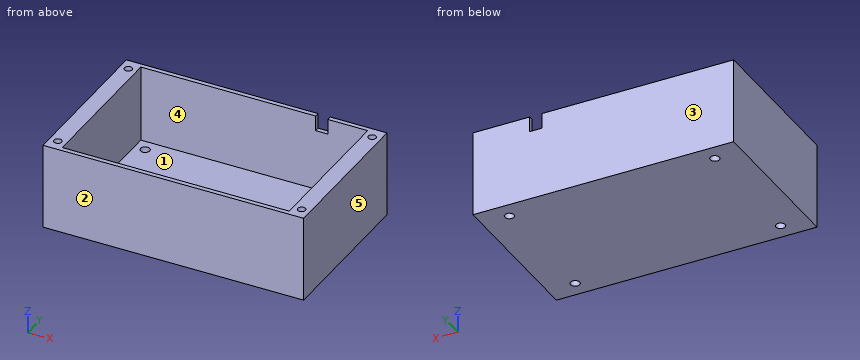
from build123d import *

# Parameters (mm, degrees)
F0_W     = 85
F0_H     = 52
F0_R     = 1.5
F1_DEPTH = 3
F2_W     = 85
F2_H     = 52
F2_W_2   = 74
F2_H_2   = 49
F3_DEPTH = 25
F4_R     = 1.25
F5_DEPTH = 10
F6_W     = 4
F6_H     = 1.5
F7_DEPTH = 5


with BuildPart() as f1:
    # F0 (on Top) → F1 (new body)
    with BuildSketch(Plane.XY):
        Rectangle(F0_W, F0_H)
        with Locations((-33.5, -20.5)):
            Circle(F0_R, mode=Mode.SUBTRACT)
        with Locations((33.5, -20.5)):
            Circle(F0_R, mode=Mode.SUBTRACT)
        with Locations((-33.5, 20.5)):
            Circle(F0_R, mode=Mode.SUBTRACT)
        with Locations((33.5, 20.5)):
            Circle(F0_R, mode=Mode.SUBTRACT)
    extrude(amount=F1_DEPTH)

    # F2 (on face) → F3 (join)
    with BuildSketch(Plane.XY.offset(3)):
        Rectangle(F2_W, F2_H)
        Rectangle(F2_W_2, F2_H_2, mode=Mode.SUBTRACT)
    extrude(amount=F3_DEPTH)

    # F4 (on face) → F5 (cut)
    with BuildSketch(Plane.XY.offset(28)):
        with Locations((-39.75, 22)):
            Circle(F4_R)
        with Locations((-39.75, -22)):
            Circle(F4_R)
        with Locations((39.75, 22)):
            Circle(F4_R)
        with Locations((39.75, -22)):
            Circle(F4_R)
    extrude(amount=-F5_DEPTH, mode=Mode.SUBTRACT)

    # F6 (on face) → F7 (cut)
    with BuildSketch(Plane.XY.offset(28)):
        with Locations((22, 25.25)):
            Rectangle(F6_W, F6_H)
    extrude(amount=-F7_DEPTH, mode=Mode.SUBTRACT)


solid = f1.part
Work out the finished part from the listing and answer in its coordinate system (mm). Face numbers are marked on the shaded views. A direction names the side the tool comes from. Give positions to 0.01 mm unless a question says otherwise; leave off trailing zeros. Order: outer loops, then holes, each group sorted by start corner. A loop starts at its lowest first (then second) coordinate and runs counter-clockwise, first axis right, second up. Notation, with made-up numbers: (0.5, 5) -> (31.5, 5) arc R33 cw to (31.5, 37) -> close; hole circle Ø9 at (72, 50.5). An arc over 180 degrees is marked (long way). Answer as a JSON object with one key per item and string values. Group by question number.
1. Flat-ended cylindrical pins translate along their axes: pin 1 Ø5 at (x, y) = (33.5, 20.5) entering from +Z; pin 2 Ø2 at (x, y) = (39.75, -22) entering from +Z; pin 3 Ø1.6 at (x, y) = (22.5, 25) entering from +Z. Find the tip coordinate at first contact, or state that the pin passes through.
2. Section B-B on x = 33.5 is taken. Determine the outline of the cut face in (y, z).
3. Consider line 1 along Y through (x, z) = (-33.5, 2.3); line 2 along Y through (x, z) = (39.75, 24.75); line 3 along Y through (x, z) = (21, 12). Determine where each line is inside the solid, lowest interval first. Write a range as [from, to].
4. Section D-D on y = -16 is taken. Determine the outline of the cut face in (x, z).
5. The mould has two halves that part along X. Classify the marked faces 3, 4 and 5: released by +X, released by -X, zero draft, split by the parting line, or undercut.
6. A tool of negligible diameter and unlimited length cuts with its end or side. For the marked faces 1 and 2, from which of +Z, -Z, +X, -X, +Y, -Y can it reach the whole face along a straight path? Write none if from no direction.
7. Section C-C on z = 19.5 is taken. Determine the outline of the cut face in (x, y), plus the area to 3 significant figures.
8. Section A-A on z = 24.5 is taken. Determine the outline of the cut face in (x, y).
Result sheet:
{
 "1": {"pin 1": "stops at z = 3", "pin 2": "stops at z = 18", "pin 3": "stops at z = 23"},
 "2": {"outline": "(-26, 0) -> (-22, 0) -> (-22, 3) -> (-24.5, 3) -> (-24.5, 28) -> (-26, 28) -> close; (-19, 0) -> (19, 0) -> (19, 3) -> (-19, 3) -> close; (22, 0) -> (26, 0) -> (26, 28) -> (24.5, 28) -> (24.5, 3) -> (22, 3) -> close"},
 "3": {"line 1": "y = [-26, -22], [-19, 19], [22, 26]", "line 2": "y = [-26, -23.25], [-20.75, 20.75], [23.25, 26]", "line 3": "y = [-26, -24.5], [24.5, 26]"},
 "4": {"outline": "(-42.5, 0) -> (42.5, 0) -> (42.5, 28) -> (37, 28) -> (37, 3) -> (-37, 3) -> (-37, 28) -> (-42.5, 28) -> close"},
 "5": {"face 3": "zero draft", "face 4": "undercut", "face 5": "released by +X"},
 "6": {"face 1": "+Z", "face 2": "+Z, -Z, +X, -X, -Y"},
 "7": {"outline": "(-42.5, -26) -> (42.5, -26) -> (42.5, 26) -> (-42.5, 26) -> close; hole circle Ø2.5 at (-39.75, -22); hole circle Ø2.5 at (-39.75, 22); hole (-37, -24.5) -> (37, -24.5) -> (37, 24.5) -> (-37, 24.5) -> close; hole circle Ø2.5 at (39.75, -22); hole circle Ø2.5 at (39.75, 22)", "area": "774 mm^2"},
 "8": {"outline": "(-42.5, -26) -> (42.5, -26) -> (42.5, 26) -> (24, 26) -> (24, 24.5) -> (37, 24.5) -> (37, -24.5) -> (-37, -24.5) -> (-37, 24.5) -> (20, 24.5) -> (20, 26) -> (-42.5, 26) -> close; hole circle Ø2.5 at (-39.75, -22); hole circle Ø2.5 at (-39.75, 22); hole circle Ø2.5 at (39.75, -22); hole circle Ø2.5 at (39.75, 22)"}
}
